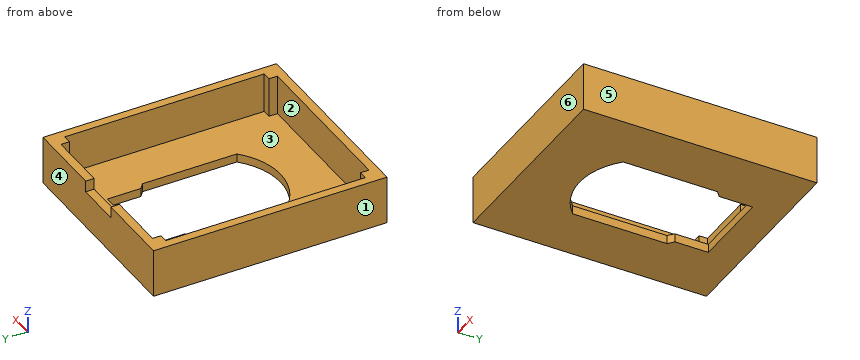
```python
from build123d import *

# Parameters (mm, degrees)
SKETCH_1_W          = 35
SKETCH_1_H          = 41
EXTRUDE_1_DEPTH     = 1.5
EXTRUDE_2_DEPTH     = 7
SKETCH_3_W          = 8
SKETCH_3_H          = 1.5
CUT_EXTRUDE_1_DEPTH = 2


with BuildPart() as part:
    # Эскиз1 → Бобышка-Вытянуть1 (new body)
    with BuildSketch(Plane.XY):
        Rectangle(SKETCH_1_W, SKETCH_1_H)
        with BuildLine():
            Line((7, 9.124143795), (7, 15))
            Line((7, 15), (-7, 15))
            Line((-7, 15), (-7, 9.124143795))
            ThreePointArc((-7, 9.124143795), (-7.512396473, 8.707117734), (-8, 8.261355821))
            Line((-8, 8.261355821), (-8, -8.261355821))
            ThreePointArc((-8, -8.261355821), (0, -11.5), (8, -8.261355821))
            Line((8, -8.261355821), (8, 8.261355821))
            ThreePointArc((8, 8.261355821), (7.512396473, 8.707117734), (7, 9.124143795))
        make_face(mode=Mode.SUBTRACT)
    extrude(amount=EXTRUDE_1_DEPTH)

    # Эскиз2 → Бобышка-Вытянуть2 (add)
    with BuildSketch(Plane.XY.offset(1.5)):
        Polygon((-17.5, -20.5), (17.5, -20.5), (17.5, 20.5), (-14.5, 20.5), (-17.5, 20.5), (-17.5, 17.5), align=None)
        Polygon((14.5, -17.5), (14.5, -19), (-14.5, -19), (-14.5, -17.5), (-16, -17.5), (-16, 17.5), (-14.5, 17.5), (-14.5, 19), (14.5, 19), (14.5, 17.5), (16, 17.5), (16, -17.5), align=None, mode=Mode.SUBTRACT)
    extrude(amount=EXTRUDE_2_DEPTH)

    # Эскиз3 → Вырез-Вытянуть1 (cut)
    with BuildSketch(Plane.XY.offset(8.5)):
        with Locations((0, 19.75)):
            Rectangle(SKETCH_3_W, SKETCH_3_H)
    extrude(amount=-CUT_EXTRUDE_1_DEPTH, mode=Mode.SUBTRACT)


solid = part.part
```
The model under review builds one solid part; all positions refer to its coordinate system, in mm. Face numbers are marked on the shaded views. A direction names the side the tool comes from. Coordinates: 2 decimals unless noted, no trailing zeros. Order: outer loops, then holes, each group sorted by start corner. A loop starts at its lowest first (then second) coordinate and runs counter-clockwise, first axis right, second up. Notation, with made-up numbers: (21, 78.25) -> (48, 78.25) arc R21 cw to (48, 100.25) -> close; hole circle Ø1 at (49.25, -23). An arc over 180 degrees is marked (long way). Answer in a Markdown table with one row per item. Add a question column.
Item 1: We need section C-C on x = -10.5. Write out the cut boundary in (y, z), plus the area to 3 significant figures.
Item 2: Clearance check with flat-ended pins moving along their axes: pin 1 (5 mm diameter, centred on x = 9, y = 12.5, fed in from +Z); pin 2 (3 mm diameter, centred on x = -5.5, y = -4.5, fed in from +Z). State where each tip first meets the part, or that it passes through.
Item 3: We need section A-A on y = -5. Write out the cut boundary in (x, z), plus the area to 3 significant figures.
Item 4: To check wall thickness, follow probe 1 along Y at (x, z) = (14, 3); probe 2 along X at (y, z) = (3, 6); probe 3 along Z at (x, y) = (-14, -8). State the ranges of each line that lie inside material, in increasing order.
Item 5: Mouldability with a two-part tool opening along Y and no side actions: class the marked faces 3, 4, 5 and 6 as +Y half, -Y half, draft (parallel to the pull), parting line (faces both ways), or undercut.
Item 6: We need section B-B on z = 4.5. Write out the cut boundary in (x, y), plus the area to 3 significant figures.
Item 7: We need section D-D on z = 7.25. Write out the cut boundary in (x, y).
Item 8: Machinability: for the marked faces 1 and 2, which of the approach directions +Z, -Z, +X, -X, +Y, -Y give a long, thin tool a straight path to every point of the face, cutting with its end or side? Answer none if there is none.
Final values:
| question | item | result |
|---|---|---|
| 1 | outline | (-20.5, 0) -> (20.5, 0) -> (20.5, 8.5) -> (19, 8.5) -> (19, 1.5) -> (-19, 1.5) -> (-19, 8.5) -> (-20.5, 8.5) -> close |
| 1 | area | 82.5 mm2 |
| 2 | pin 1 | stops at z = 1.5 |
| 2 | pin 2 | passes through |
| 3 | outline | (-17.5, 0) -> (-8, 0) -> (-8, 1.5) -> (-16, 1.5) -> (-16, 8.5) -> (-17.5, 8.5) -> close; (8, 0) -> (17.5, 0) -> (17.5, 8.5) -> (16, 8.5) -> (16, 1.5) -> (8, 1.5) -> close |
| 3 | area | 49.5 mm2 |
| 4 | probe 1 | y = -20.5 to -19, 19 to 20.5 |
| 4 | probe 2 | x = -17.5 to -16, 16 to 17.5 |
| 4 | probe 3 | z = 0 to 1.5 |
| 5 | face 3 | undercut |
| 5 | face 4 | +Y half |
| 5 | face 5 | draft |
| 5 | face 6 | -Y half |
| 6 | outline | (-17.5, -20.5) -> (17.5, -20.5) -> (17.5, 20.5) -> (-17.5, 20.5) -> close; hole (-16, -17.5) -> (-14.5, -17.5) -> (-14.5, -19) -> (14.5, -19) -> (14.5, -17.5) -> (16, -17.5) -> (16, 17.5) -> (14.5, 17.5) -> (14.5, 19) -> (-14.5, 19) -> (-14.5, 17.5) -> (-16, 17.5) -> close |
| 6 | area | 228 mm2 |
| 7 | outline | (-17.5, -20.5) -> (17.5, -20.5) -> (17.5, 20.5) -> (4, 20.5) -> (4, 19) -> (14.5, 19) -> (14.5, 17.5) -> (16, 17.5) -> (16, -17.5) -> (14.5, -17.5) -> (14.5, -19) -> (-14.5, -19) -> (-14.5, -17.5) -> (-16, -17.5) -> (-16, 17.5) -> (-14.5, 17.5) -> (-14.5, 19) -> (-4, 19) -> (-4, 20.5) -> (-17.5, 20.5) -> close |
| 8 | face 1 | +Z, -Z, -X, +Y, -Y |
| 8 | face 2 | +Z |
